The listing builds one solid part. Answer for the finished solid, in the listing's coordinates (mm). Give positions to 0.01 mm unless a question says otherwise; leave off trailing zeros. Write each loop counter-clockwise with the first axis right and the second up, starting at its lowest first coordinate (ties: lowest second). Pieces come first, ordered by that corner, then holes.
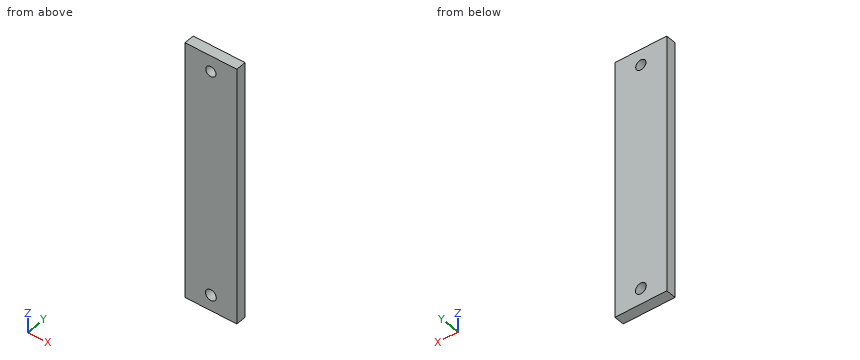
Autodesk Inventor part; units mm, degrees
ref_plane "YZ Plane" through (0, 0, 0) normal (1, 0, 0) x (0, 1, 0)
ref_plane "XZ Plane" through (0, 0, 0) normal (0, 1, 0) x (-1, 0, 0)
ref_plane "XY Plane" through (0, 0, 0) normal (0, 0, 1) x (1, 0, 0)
sketch "Sketch1" plane through (0, 0, 0) normal (0, 1, 0) x (-1, 0, 0)
  line L0 (0, 0) -> (-127, 0)
  line L1 (-127, 0) -> (-127, -635)
  line L2 (-127, -635) -> (0, -635)
  line L3 (0, -635) -> (0, 0)
  circle A0 centre (-63.5, -38.9382) radius 12.5273
  circle A1 centre (-63.5, -596.0618) radius 13.2642
  dimension "d0" = 127
  dimension "d1" = 635
  dimension "d2" = 38.9382
  dimension "d3" = 38.9382
extrude "Extrusion1" add sketch "Sketch1" along normal blind 25.4
properties part number "Frame"
Item 1: Consider probe 1 along Z at (x, y) = (63.5, 18.75); probe 2 along Z at (x, y) = (64.5, 19.5). Determine where each line is inside the solid, lowest interval first.
Conclusion:
probe 1: z = -635 to -609.33, -582.8 to -51.47, -26.41 to 0
probe 2: z = -635 to -609.29, -582.84 to -51.43, -26.45 to 0
Item 2: This flat-tipped pin is pushed along its axis until it touches: P1, Ø5, axis at x = 75.5, y = 10, coming from the +Z side. Where does it stop, or does it pass through?
Conclusion:
P1: stops at z = 0
Item 3: A cutting plane is placed at A-A, the plane x = 63.5. Give the vertices of the cut face in (y, z), plus the area to 3 significant figures.
Conclusion:
outline: (0, -635) - (25.4, -635) - (25.4, -609.33) - (0, -609.33) - close; (0, -582.8) - (25.4, -582.8) - (25.4, -51.47) - (0, -51.47) - close; (0, -26.41) - (25.4, -26.41) - (25.4, 0) - (0, 0) - close
area: 14,800 mm2
